Check sheet for the modelled part. Datum: model origin and axes. Units: mm. A direction names the side the tool comes from. Round coordinates to 2 decimals unless told otherwise and drop trailing zeros. Order: outer loops, then holes, each group sorted by start corner. A loop starts at its lowest first (then second) coordinate and runs counter-clockwise, first axis right, second up. Notation, with made-up numbers: (38.5, 67.5) -> (67.5, 67.5) arc R37 ccw to (67.5, 103.5) -> close; hole circle Ø3 at (27, 61.5). An arc over 180 degrees is marked (long way). Answer in a Markdown table with one row per item.
```python
from build123d import *

# Parameters (mm, degrees)
SKETCH6_R           = 2.5
BOSS_EXTRUDE2_DEPTH = 3
SKETCH7_R           = 3
CUT_EXTRUDE2_DEPTH  = 16


with BuildPart() as part:
    # Sketch4 → Revolve1 (revolve)
    with BuildSketch(Plane.XY):
        Polygon((-7.5, 15), (7.5, 15), (7.5, 20), (9, 20), (9, 0), (-9, 0), (-9, 20), (-7.5, 20), align=None)
    revolve(axis=Axis((9, 0, 0), (-1, 0, 0)))

    # Sketch6 → Boss-Extrude2 (add)
    with BuildSketch(Plane(origin=(9, 0, 0), x_dir=(0, 0, -1), z_dir=(1, 0, 0))):
        with Locations(Location((0, 13.5, 0), (0, 0, 90))):
            Circle(SKETCH6_R)
    extrude(amount=BOSS_EXTRUDE2_DEPTH)

    # Sketch7 → Cut-Extrude2 (cut)
    with BuildSketch(Plane.ZY.offset(9)):
        with Locations(Location((0, 0, 0), (0, 0, 270))):
            Circle(SKETCH7_R)
    extrude(amount=-CUT_EXTRUDE2_DEPTH, mode=Mode.SUBTRACT)


solid = part.part
```
(1) Tool access check on faces 1 (the flat face through (-7.5, 3, -15)), 2 (the cylindrical face through (-8.24, -4.336, 19.524)), 3 (the flat face through (7, 0, 0)). Record the directions out of +Z, -Z, +X, -X, +Y, -Y that give a thin tool (end or side, any length) a straight path to the whole face; none if there is none.
Solutions:
| item | result |
|---|---|
| face 1 | none |
| face 2 | +X, -X |
| face 3 | -X |
(2) Section check A-A on y = 12. Record the boundary of the cut face in (x, z), plus the area to 3 significant figures.
Solutions:
| item | result |
|---|---|
| outline | (-9, -16) -> (-7.5, -16) -> (-7.5, -9) -> (7.5, -9) -> (7.5, -16) -> (9, -16) -> (9, -2) -> (12, -2) -> (12, 2) -> (9, 2) -> (9, 16) -> (7.5, 16) -> (7.5, 9) -> (-7.5, 9) -> (-7.5, 16) -> (-9, 16) -> close |
| area | 378 mm^2 |
(3) Section check B-B on z = 0. Record the boundary of the cut face in (x, y).
Solutions:
| item | result |
|---|---|
| outline | (-9, -20) -> (-7.5, -20) -> (-7.5, -15) -> (7.5, -15) -> (7.5, -20) -> (9, -20) -> (9, 11) -> (12, 11) -> (12, 16) -> (9, 16) -> (9, 20) -> (7.5, 20) -> (7.5, 15) -> (-7.5, 15) -> (-7.5, 20) -> (-9, 20) -> (-9, 3) -> (7, 3) -> (7, -3) -> (-9, -3) -> close |
(4) Scan lines: probe 1 along Z at (x, y) = (3, 0); probe 2 along X at (y, z) = (-16, 2); probe 3 along Z at (x, y) = (-2, 12). Record each from-to range of solid material in increasing order. Write a range as from..to.
Solutions:
| item | result |
|---|---|
| probe 1 | -15..-3, 3..15 |
| probe 2 | -9..-7.5, 7.5..9 |
| probe 3 | -9..9 |
(5) Section check D-D on x = 8. Record the boundary of the cut face in (y, z), plus the area to 3 significant figures.
Solutions:
| item | result |
|---|---|
| outline | circle Ø40 at (0, 0) |
| area | 1,260 mm^2 |
(6) Section check C-C on z = 15.5. Record the boundary of the cut face in (x, y), plus the area to 3 significant figures.
Solutions:
| item | result |
|---|---|
| outline | (-9, -12.64) -> (-7.5, -12.64) -> (-7.5, 12.64) -> (-9, 12.64) -> close; (7.5, -12.64) -> (9, -12.64) -> (9, 12.64) -> (7.5, 12.64) -> close |
| area | 75.8 mm^2 |
(7) Draft check along Y on faces 4 (the cylindrical face through (10, 11, 0)), 5 (the flat face through (7.5, -3, -15)), 6 (the cylindrical face through (-1.11, -2.86, 0.9)). Enter one of: pulls with the +Y half, pulls with the -Y half, needs draft (parallel to the pull), parting line crosses it, or undercut.
Solutions:
| item | result |
|---|---|
| face 4 | parting line crosses it |
| face 5 | needs draft |
| face 6 | undercut |
(8) Depth check by flat-ended pin: pin 1 Ø8 at (x, y) = (-6.5, 10.5) entering from -Z; pin 2 Ø6 at (x, y) = (2, 4) entering from +Z; pin 3 Ø1 at (x, y) = (8, -12) entering from -Z. Enter the tip coordinate at first touch or a pass-through.
Solutions:
| item | result |
|---|---|
| pin 1 | z = -18.87 |
| pin 2 | z = 14.97 |
| pin 3 | z = -16.36 |
